Geometry check sheet. Reference: the model listing, model coordinates, mm. A direction names the side the tool comes from. Give positions to 0.01 mm unless a question says otherwise; leave off trailing zeros. Order: outer loops, then holes, each group sorted by start corner. A loop starts at its lowest first (then second) coordinate and runs counter-clockwise, first axis right, second up. Notation, with made-up numbers: M -38.5,24.5 L 0.5,24.5 A22 cw 0.5,42.5 Z; hole C -27.5,44.25 d11. An arc over 180 degrees is marked long. Put each result on its own line as item: value. Start each with the question number.
Q1. Access from +Z, -Z, +X, -X, +Y, -Y to the whole of each face (thin tool, end or side, straight path). Record for faces 1 (the cylindrical face through (19.1, 9.14, -17.32)), 2 (the cylindrical face through (-19.1, 9.14, -17.68)), 3 (the flat face through (0, 10, -19)), 4 (the flat face through (0, -10, -19)).
Q2. Material ranges on L1, parallel to X at y = 0.75, z = -30; L2, parallel to Z at x = -0.5, y = 5.75; L3, parallel to Y at x = 3.5, z = -43.5, recorded low to high.
Q3. Section check B-B on y = -8.5. Record the cut outline in (x, z).
Q4. Section check A-A on x = 0. Record the cut outline in (y, z).
Q5. Go/stop test with flat-tipped pins: pin 1 (2 mm diameter, centred on y = 9.5, z = -7.5, fed in from +X); pin 2 (2 mm diameter, centred on y = 0.5, z = 1.5, fed in from +X); pin 3 (4 mm diameter, centred on y = -2.5, z = -14.5, fed in from +X); pin 4 (2 mm diameter, centred on x = 22.5, z = -14.5, fed in from +Y). Record where each tip stops, or that it passes through.
Q6. Section check C-C on y = 12.75. Record the cut outline in (x, z).
```python
from build123d import *

# Parameters (mm, degrees)
SKETCH1_W           = 60
SKETCH1_H           = 30
BOSS_EXTRUDE1_DEPTH = 15
SKETCH2_R           = 10
BOSS_EXTRUDE2_DEPTH = 10
FILLET1_R           = 5
FILLET2_R           = 3


with BuildPart() as part:
    # Sketch1 → Boss-Extrude1 (new body)
    with BuildSketch(Plane.XY):
        Rectangle(SKETCH1_W, SKETCH1_H)
    extrude(amount=BOSS_EXTRUDE1_DEPTH)

    # Sketch2 → Boss-Extrude2 (add, symmetric)
    with BuildSketch(Plane(origin=(0, 0, 0), x_dir=(1, 0, 0), z_dir=(0, 1, 0))):
        with BuildLine():
            Line((-20, 30), (-20, 0))
            Line((-20, 0), (20, 0))
            Line((20, 0), (20, 30))
            ThreePointArc((20, 30), (0, 50), (-20, 30))
        make_face()
        with Locations(Location((0, 30, 0), (0, 0, 270))):
            Circle(SKETCH2_R, mode=Mode.SUBTRACT)
    extrude(amount=BOSS_EXTRUDE2_DEPTH, both=True)

    # Fillet1
    fillet1_edges = [part.edges().sort_by_distance(p)[0] for p in [
        (-20, 0, 0),
        (20, 0, 0),
    ]]
    fillet(fillet1_edges, radius=FILLET1_R)

    # Fillet2
    # the kernel refuses this fillet: 3 mm, written as the material it takes off along each edge
    with BuildSketch(Plane(origin=(0, 10, -30), x_dir=(1, 0, 0), z_dir=(0, 0, 1))) as fillet2_piece_1:
        with BuildLine():
            CenterArc((20 - FILLET2_R, -FILLET2_R), FILLET2_R, 0, 90)
            Line((20 - FILLET2_R, 0), (20, 0))
            Line((20, 0), (20, -FILLET2_R))
        make_face()
    revolve(axis=Axis((0, 10, -30), (0, 1, 0)), revolution_arc=180, mode=Mode.SUBTRACT)
    with BuildSketch(Plane(origin=(-20, 10, -30), x_dir=(0, -1, 0), z_dir=(0, 0, 1)), Plane(origin=(20, 10, -5), x_dir=(0, -1, 0), z_dir=(0, 0, -1))) as fillet2_piece_2:
        with BuildLine():
            CenterArc((FILLET2_R, FILLET2_R), FILLET2_R, 180, 90)
            Line((0, FILLET2_R), (0, 0))
            Line((0, 0), (FILLET2_R, 0))
        make_face()
    extrude(amount=25, mode=Mode.SUBTRACT)
    with BuildSketch(Plane(origin=(0, -10, -30), x_dir=(1, 0, 0), z_dir=(0, 0, 1))) as fillet2_piece_3:
        with BuildLine():
            CenterArc((20 - FILLET2_R, FILLET2_R), FILLET2_R, 270, 90)
            Line((20 - FILLET2_R, 0), (20, 0))
            Line((20, 0), (20, FILLET2_R))
        make_face()
    revolve(axis=Axis((0, -10, -30), (0, 1, 0)), revolution_arc=180, mode=Mode.SUBTRACT)
    with BuildSketch(Plane(origin=(-20, -10, -30), x_dir=(0, 1, 0), z_dir=(0, 0, 1)), Plane(origin=(20, -10, -5), x_dir=(0, 1, 0), z_dir=(0, 0, -1))) as fillet2_piece_4:
        with BuildLine():
            CenterArc((FILLET2_R, -FILLET2_R), FILLET2_R, 90, 90)
            Line((0, -FILLET2_R), (0, 0))
            Line((0, 0), (FILLET2_R, 0))
        make_face()
    extrude(amount=25, mode=Mode.SUBTRACT)
    with BuildSketch(Plane(origin=(25, -10, -5), x_dir=(0.9975374290817743, 0, 0.07013613605641604), z_dir=(0.07013613605641604, 0, -0.9975374290817743))) as fillet2_piece_5_section:
        with BuildLine():
            CenterArc((5 + FILLET2_R, -FILLET2_R), FILLET2_R, 90, 90)
            Line((5 + FILLET2_R, 0), (5, 0))
            Line((5, 0), (5, -FILLET2_R))
        make_face()
    fillet2_piece_5 = revolve(axis=Axis((25, -10, -5), (0, -1, 0)), revolution_arc=175.978193542, mode=Mode.PRIVATE)
    fillet2_piece_5 = split(fillet2_piece_5, bisect_by=Plane(origin=(21.314130097, -9.156886231, 0), z_dir=(0, 0, -1)), keep=Keep.TOP, mode=Mode.PRIVATE)
    add(fillet2_piece_5, mode=Mode.SUBTRACT)
    with BuildSketch(Plane(origin=(25, 10, -5), x_dir=(0.9975374290817743, 0, 0.07013613605641604), z_dir=(0.07013613605641604, 0, -0.9975374290817743))) as fillet2_piece_6_section:
        with BuildLine():
            CenterArc((5 + FILLET2_R, FILLET2_R), FILLET2_R, 180, 90)
            Line((5, FILLET2_R), (5, 0))
            Line((5, 0), (5 + FILLET2_R, 0))
        make_face()
    fillet2_piece_6 = revolve(axis=Axis((25, 10, -5), (0, -1, 0)), revolution_arc=175.978193542, mode=Mode.PRIVATE)
    fillet2_piece_6 = split(fillet2_piece_6, bisect_by=Plane(origin=(21.314129988, 9.156886191, 0), z_dir=(0, 0, -1)), keep=Keep.TOP, mode=Mode.PRIVATE)
    add(fillet2_piece_6, mode=Mode.SUBTRACT)
    with BuildSketch(Plane(origin=(-25, -10, -5), x_dir=(-0.9975374290817743, 0, 0.07013613605641587), z_dir=(-0.07013613605641587, 0, -0.9975374290817743))) as fillet2_piece_7_section:
        with BuildLine():
            CenterArc((5 + FILLET2_R, FILLET2_R), FILLET2_R, 180, 90)
            Line((5 + FILLET2_R, 0), (5, 0))
            Line((5, 0), (5, FILLET2_R))
        make_face()
    fillet2_piece_7 = revolve(axis=Axis((-25, -10, -5), (0, 1, 0)), revolution_arc=175.978193542, mode=Mode.PRIVATE)
    fillet2_piece_7 = split(fillet2_piece_7, bisect_by=Plane(origin=(-21.314129744, -9.156885957, 0), z_dir=(0, 0, -1)), keep=Keep.TOP, mode=Mode.PRIVATE)
    add(fillet2_piece_7, mode=Mode.SUBTRACT)
    with BuildSketch(Plane(origin=(-25, 10, -5), x_dir=(-0.9975374290817743, 0, 0.07013613605641587), z_dir=(-0.07013613605641587, 0, -0.9975374290817743))) as fillet2_piece_8_section:
        with BuildLine():
            CenterArc((5 + FILLET2_R, -FILLET2_R), FILLET2_R, 90, 90)
            Line((5 + FILLET2_R, 0), (5, 0))
            Line((5, 0), (5, -FILLET2_R))
        make_face()
    fillet2_piece_8 = revolve(axis=Axis((-25, 10, -5), (0, 1, 0)), revolution_arc=175.978193542, mode=Mode.PRIVATE)
    fillet2_piece_8 = split(fillet2_piece_8, bisect_by=Plane(origin=(-21.314129744, 9.156885957, 0), z_dir=(0, 0, -1)), keep=Keep.TOP, mode=Mode.PRIVATE)
    add(fillet2_piece_8, mode=Mode.SUBTRACT)
    with BuildSketch(Plane(origin=(37.5, -15, 0), x_dir=(0, 1, 0), z_dir=(-1, 0, 0)), Plane(origin=(-37.5, 15, 0), x_dir=(0, -1, 0), z_dir=(1, 0, 0))) as fillet2_piece_9:
        with BuildLine():
            CenterArc((FILLET2_R, -FILLET2_R), FILLET2_R, 90, 90)
            Line((0, -FILLET2_R), (0, 0))
            Line((0, 0), (FILLET2_R, 0))
        make_face()
    extrude(amount=75, mode=Mode.SUBTRACT)
    with BuildSketch(Plane(origin=(-30, -22.5, 0), x_dir=(1, 0, 0), z_dir=(0, 1, 0)), Plane(origin=(30, 22.5, 0), x_dir=(-1, 0, 0), z_dir=(0, -1, 0))) as fillet2_piece_10:
        with BuildLine():
            CenterArc((FILLET2_R, -FILLET2_R), FILLET2_R, 90, 90)
            Line((0, -FILLET2_R), (0, 0))
            Line((0, 0), (FILLET2_R, 0))
        make_face()
    extrude(amount=45, mode=Mode.SUBTRACT)


solid = part.part
```
Results found:
1. face 1: -Z, +X, +Y
1. face 2: -Z, -X, +Y
1. face 3: -Z, +X, -X, +Y
1. face 4: -Z, +X, -X, -Y
2. L1: x = -20 to -10, 10 to 20
2. L2: z = -49.99 to -39.99, -20.01 to 15
2. L3: y = -10 to 10
3. outline: M -30,3 A3 ccw -27,0 L -22.96,0 A5.4 cw -19.6,-5 L -19.6,-30 A19.6 ccw 19.6,-30 L 19.6,-5 A5.4 cw 22.96,0 L 27,0 A3 ccw 30,3 L 30,15 L -30,15 Z; hole C 0,-30 d20
4. outline: M -15,3 A3 ccw -12,0 L -10,0 L -10,-20 L 10,-20 L 10,0 L 12,0 A3 ccw 15,3 L 15,15 L -15,15 Z; M -10,-47 A3 ccw -7,-50 L 7,-50 A3 ccw 10,-47 L 10,-40 L -10,-40 Z
5. pin 1: stops at x = 19.6
5. pin 2: stops at x = 29.96
5. pin 3: stops at x = 20
5. pin 4: passes through
6. outline: M -30,3 A3 ccw -27.75,0.1 L 27.75,0.1 A3 ccw 30,3 L 30,15 L -30,15 Z
